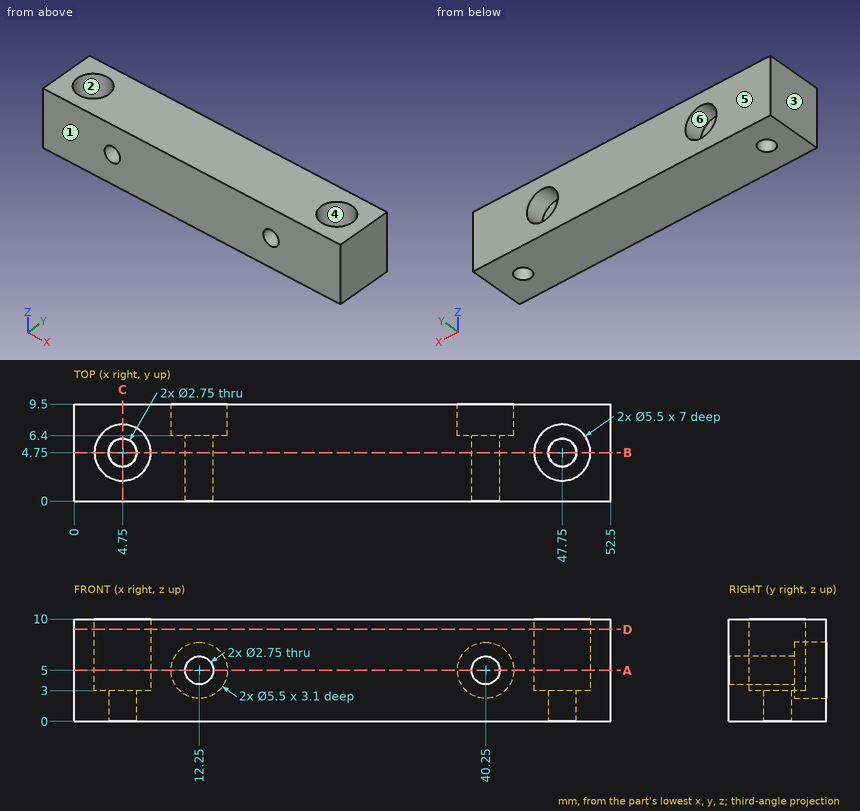
Source: three-view drawing plus pictorial views. Frame: mm from the lowest corner of the part. A direction names the side the tool comes from. Round coordinates to 2 decimals unless told otherwise and drop trailing zeros. Loops run counter-clockwise (first coordinate to the right, second up) from the corner with the lowest first, then second, coordinate; pieces in that order, holes last. Notation, with made-up numbers: M -15,10 L 37,10 A17 ccw 37,36 Z; hole C 87.25,-12 d7. An arc over 180 degrees is marked long. Put each result on its own line as item: value. Start each with the question number.
(1) Set-up query: the marked faces 4, 5 and 6. Return all of +Z, -Z, +X, -X, +Y, -Y with unobstructed straight access to the full face (end or side cutting, diameter ignored); none if empty.
(2) Section query B-B (y = 4.75). Return loops of the section in (x, z) (3 decimals).
(3) Section query D-D (z = 9). Return loops of the section in (x, y), then the cut area to 3 significant figures.
(4) Draft query along X for the marked faces 1, 2 and 3. Return one class per face: +X half, -X half, draft (parallel to the pull), parting line (faces both ways), or undercut.
(5) Material intervals for line 1 along X through (y, z) = (8.35, 5); line 2 along X through (y, z) = (6.25, 5.75); line 3 along X through (y, z) = (6.75, 4), sorted ascending. Write a range as [from, to].
(6) Contact query for flat-ended pins moving along their axis: pin 1 Ø3.5 at (x, y) = (4.75, 4.75) entering from +Z; pin 2 Ø4.5 at (x, z) = (12.25, 5) entering from +Y. Output: stop coordinate, or through.
(7) Section query A-A (z = 5). Return loops of the section in (x, y) (3 decimals), then the cut area to 3 significant figures.
(8) Section query C-C (x = 4.75). Return loops of the section in (y, z) (3 decimals).
Findings below:
1. face 4: +Z
1. face 5: +Z, -Z, +X, -X, +Y
1. face 6: +Y
2. outline: M 0,0 L 3.375,0 L 3.375,3 L 2,3 L 2,10 L 0,10 Z; M 6.125,0 L 46.375,0 L 46.375,3 L 45,3 L 45,10 L 7.5,10 L 7.5,3 L 6.125,3 Z; M 49.125,0 L 52.5,0 L 52.5,10 L 50.5,10 L 50.5,3 L 49.125,3 Z; hole C 12.25,5 d2.75; hole C 40.25,5 d2.75
3. outline: M 0,0 L 52.5,0 L 52.5,9.5 L 0,9.5 Z; hole C 4.75,4.75 d5.5; hole C 47.75,4.75 d5.5
3. area: 451 mm2
4. face 1: draft
4. face 2: undercut
4. face 3: -X half
5. line 1: x = [0, 9.5], [15, 37.5], [43, 52.5]
5. line 2: x = [0, 2.45], [7.05, 11.1], [13.4, 39.1], [41.4, 45.45], [50.05, 52.5]
5. line 3: x = [0, 2.86], [6.64, 9.69], [14.81, 37.69], [42.81, 45.86], [49.64, 52.5]
6. pin 1: stops at z = 3
6. pin 2: stops at y = 6.4
7. outline: M 0,0 L 10.875,0 L 10.875,6.4 L 9.5,6.4 L 9.5,9.5 L 0,9.5 Z; M 13.625,0 L 38.875,0 L 38.875,6.4 L 37.5,6.4 L 37.5,9.5 L 15,9.5 L 15,6.4 L 13.625,6.4 Z; M 41.625,0 L 52.5,0 L 52.5,9.5 L 43,9.5 L 43,6.4 L 41.625,6.4 Z; hole C 4.75,4.75 d5.5; hole C 47.75,4.75 d5.5
7. area: 382 mm2
8. outline: M 0,0 L 3.375,0 L 3.375,3 L 2,3 L 2,10 L 0,10 Z; M 6.125,0 L 9.5,0 L 9.5,10 L 7.5,10 L 7.5,3 L 6.125,3 Z
